```python
from build123d import *

# Parameters (mm, degrees)
RESSALTO_EXTRUS_O1_DEPTH    = 285
CORTE_EXTRUS_O1_DEPTH       = 286
RESSALTO_EXTRUS_O3_DEPTH    = 285
ESBO_O13_W                  = 1.5
ESBO_O13_H                  = 2
CORTE_EXTRUS_O7_DEPTH       = 52.25
CORTE_EXTRUS_O7_DEPTH_BACK  = 52.25
RESSALTO_EXTRUS_O5_DEPTH    = 10
ESBO_O5_R                   = 1.25
CORTE_EXTRUS_O3_DEPTH       = 10
ESBO_O6_W                   = 10
ESBO_O6_H                   = 6.190700041
RESSALTO_EXTRUS_O4_DEPTH    = 11
ESBO_O7_R                   = 2.25
CORTE_EXTRUS_O4_DEPTH       = 12
ESBO_O9_R                   = 1.65
CORTE_EXTRUS_O5_DEPTH       = 10
RESSALTO_EXTRUS_O6_DEPTH    = 15
ESBO_O12_R                  = 2.5
CORTE_EXTRUS_O8_DEPTH       = 20
CORTE_EXTRUS_O9_START       = -11
ESBO_O14_R                  = 6
CORTE_EXTRUS_O9_DEPTH       = 100
PADR_O_LINEAR1_COUNT        = 2
PADR_O_LINEAR1_PITCH        = 230
ESBO_O16_W                  = 118.931950447
ESBO_O16_H                  = 98.407051197
ESBO_O16_W_2                = 168.047643727
ESBO_O16_H_2                = 92.783791129
CORTE_EXTRUS_O11_DEPTH      = 55.553847577
CORTE_EXTRUS_O11_DEPTH_BACK = 55.603847577


with BuildPart() as part:
    # Esbo_o1 → Ressalto-extrus_o1 (new body)
    with BuildSketch(Plane.XY):
        Polygon((-46.053847577, 79.767603888), (-51.25, 88.767603888), (-48.82913331, 88.767603888), (-47.882520117, 115.87505904), (-45.882520117, 115.87505904), (-44.935906924, 88.767603888), (-41.435906924, 88.767603888), (-40.393073045, 118.630458973), (-38.393073045, 118.630458973), (-37.350239166, 88.767603888), (-33.850239166, 88.767603888), (-32.727930438, 120.906320886), (-30.727930438, 120.906320886), (-29.60562171, 88.767603888), (-26.10562171, 88.767603888), (-24.921032923, 122.689788425), (-22.921032923, 122.689788425), (-21.736444137, 88.767603888), (-18.236444137, 88.767603888), (-17.007119627, 123.970851902), (-15.007119627, 123.970851902), (-13.777795118, 88.767603888), (-10.277795118, 88.767603888), (-9.021529135, 124.742354757), (-7.021529135, 124.742354757), (-5.765263153, 88.767603888), (-2.265263153, 88.767603888), (-1, 125), (1, 125), (2.265263153, 88.767603888), (5.765263153, 88.767603888), (7.021529135, 124.742354757), (9.021529135, 124.742354757), (10.277795118, 88.767603888), (13.777795118, 88.767603888), (15.007119627, 123.970851902), (17.007119627, 123.970851902), (18.236444137, 88.767603888), (21.736444137, 88.767603888), (22.921032923, 122.689788425), (24.921032923, 122.689788425), (26.10562171, 88.767603888), (29.60562171, 88.767603888), (30.727930438, 120.906320886), (32.727930438, 120.906320886), (33.850239166, 88.767603888), (37.350239166, 88.767603888), (38.393073045, 118.630458973), (40.393073045, 118.630458973), (41.435906924, 88.767603888), (44.935906924, 88.767603888), (45.882520117, 115.87505904), (47.882520117, 115.87505904), (48.82913331, 88.767603888), (51.25, 88.767603888), (46.053847577, 79.767603888), align=None)
    extrude(amount=RESSALTO_EXTRUS_O1_DEPTH)

    # Esbo_o2 → Corte-extrus_o1 (cut, through all)
    with BuildSketch(Plane.XY.offset(285)):
        Polygon((-47.003847577, 81.413052155), (-43.972758664, 83.163052155), (-45.072758664, 85.068308043), (-48.103847577, 83.318308043), align=None)
    extrude(amount=-CORTE_EXTRUS_O1_DEPTH, mode=Mode.SUBTRACT)


with BuildPart() as body_2:
    # Esbo_o3 → Ressalto-extrus_o3 (new body)
    with BuildSketch(Plane.XY.offset(285)):
        Polygon((47.053847577, 81.499654695), (48.053847577, 83.231705503), (49.785898385, 82.231705503), (48.785898385, 80.499654695), align=None)
    extrude(amount=-RESSALTO_EXTRUS_O3_DEPTH)


with BuildPart() as corte_extrus_o7_tool:
    # Esbo_o13 → Corte-extrus_o7 (new body, two sides)
    with BuildSketch(Plane(origin=(0, 0, 0), x_dir=(0, 0, -1), z_dir=(1, 0, 0))) as corte_extrus_o7_sk:
        with Locations((-284.25, 82.767603888)):
            Rectangle(ESBO_O13_W, ESBO_O13_H)
    extrude(amount=CORTE_EXTRUS_O7_DEPTH)
    extrude(corte_extrus_o7_sk.sketch, amount=-CORTE_EXTRUS_O7_DEPTH_BACK)


with BuildPart() as part_1:
    add(part.part)

    # Corte-extrus_o7: cut by corte_extrus_o7_tool
    add(corte_extrus_o7_tool.part, mode=Mode.SUBTRACT)



with BuildPart() as body_2_1:
    add(body_2.part)

    # Corte-extrus_o7: cut by corte_extrus_o7_tool
    add(corte_extrus_o7_tool.part, mode=Mode.SUBTRACT)


with BuildPart() as part_2:
    add(part_1.part)

    add(body_2_1.part)  # Ressalto-extrus_o5 merges body 2
    # Esbo_o8 → Ressalto-extrus_o5 (add)
    with BuildSketch(Plane(origin=(0, 0, 0), x_dir=(0, 0, -1), z_dir=(0.866025404, -0.5, 0))):
        with BuildLine():
            Line((-280, 104.107695155), (-280, 96.107695155))
            Line((-280, 96.107695155), (-270, 96.107695155))
            Line((-270, 96.107695155), (-270, 104.107695155))
            ThreePointArc((-270, 104.107695155), (-275, 109.107695155), (-280, 104.107695155))
        make_face()
    ressalto_extrus_o5 = extrude(amount=-RESSALTO_EXTRUS_O5_DEPTH)

    # Esbo_o5 → Corte-extrus_o3 (cut)
    with BuildSketch(Plane.XY.offset(285)):
        with Locations((-30, 85.267603888)):
            Circle(ESBO_O5_R)
        with Locations((30, 85.267603888)):
            Circle(ESBO_O5_R)
    extrude(amount=-CORTE_EXTRUS_O3_DEPTH, mode=Mode.SUBTRACT)

    # Esbo_o6 → Ressalto-extrus_o4 (add)
    with BuildSketch(Plane(origin=(0, 0, 0), x_dir=(0, 0, 1), z_dir=(-0.866025404, -0.5, 0))):
        with BuildLine():
            Line((280, 102.5), (280, 104.207693629))
            ThreePointArc((280, 104.207693629), (275, 109.207695155), (270, 104.207693629))
            Line((270, 104.207693629), (270, 102.5))
            Line((270, 102.5), (280, 102.5))
        make_face()
        with Locations((275, 99.404649979)):
            Rectangle(ESBO_O6_W, ESBO_O6_H)
    ressalto_extrus_o4 = extrude(amount=-RESSALTO_EXTRUS_O4_DEPTH)

    # Esbo_o7 → Corte-extrus_o4 (cut)
    with BuildSketch(Plane(origin=(0, 0, 0), x_dir=(0, 0, 1), z_dir=(-0.866025404, -0.5, 0))):
        with Locations((275, 104.207695155)):
            Circle(ESBO_O7_R)
    corte_extrus_o4 = extrude(amount=-CORTE_EXTRUS_O4_DEPTH, mode=Mode.SUBTRACT)

    # Esbo_o9 → Corte-extrus_o5 (cut)
    with BuildSketch(Plane(origin=(0, 0, 0), x_dir=(0, 0, -1), z_dir=(0.866025404, -0.5, 0))):
        with Locations((-275, 104.107695155)):
            Circle(ESBO_O9_R)
    corte_extrus_o5 = extrude(amount=-CORTE_EXTRUS_O5_DEPTH, mode=Mode.SUBTRACT)

    # Esbo_o10 → Ressalto-extrus_o6 (add)
    with BuildSketch(Plane(origin=(0, 0, 0), x_dir=(-1, 0, 0), z_dir=(0, 0, -1))):
        Polygon((5.765263153, 88.767603888), (6.680885729, 114.987603888), (1.349640577, 114.987603888), (2.265263153, 88.767603888), align=None)
        Polygon((-2.265263153, 88.767603888), (-1.349640577, 114.987603888), (-6.680885729, 114.987603888), (-5.765263153, 88.767603888), align=None)
    extrude(amount=-RESSALTO_EXTRUS_O6_DEPTH)

    # Esbo_o12 → Corte-extrus_o8 (cut)
    with BuildSketch(Plane(origin=(0, 0, 0), x_dir=(-1, 0, 0), z_dir=(0, 0, -1))):
        with Locations((0, 104.999999962)):
            Circle(ESBO_O12_R)
    extrude(amount=-CORTE_EXTRUS_O8_DEPTH, mode=Mode.SUBTRACT)

    # Esbo_o14 → Corte-extrus_o9 (cut)
    with BuildSketch(Plane(origin=(0, 0, 0), x_dir=(0, 0, 1), z_dir=(-0.866025404, -0.5, 0)).offset(CORTE_EXTRUS_O9_START)):
        with Locations((275, 104.207695155)):
            Circle(ESBO_O14_R)
    corte_extrus_o9 = extrude(amount=-CORTE_EXTRUS_O9_DEPTH, mode=Mode.SUBTRACT)

    # Padr_o linear1: Ressalto-extrus_o5, Ressalto-extrus_o4, Corte-extrus_o4, Corte-extrus_o5, Corte-extrus_o9 ×2
    with Locations(*[(0, 0, -i * PADR_O_LINEAR1_PITCH) for i in range(1, PADR_O_LINEAR1_COUNT)]):
        add(ressalto_extrus_o5)
        add(ressalto_extrus_o4)
        add(corte_extrus_o4, mode=Mode.SUBTRACT)
        add(corte_extrus_o5, mode=Mode.SUBTRACT)
        add(corte_extrus_o9, mode=Mode.SUBTRACT)

    # Esbo_o16 → Corte-extrus_o11 (cut, two sides)
    with BuildSketch(Plane(origin=(0, 0, 0), x_dir=(0, 0, -1), z_dir=(1, 0, 0))) as corte_extrus_o11_sk:
        with Locations((-250.695007134, 104.881737693)):
            Rectangle(ESBO_O16_W, ESBO_O16_H)
        with Locations((-57.205210046, 102.070107659)):
            Rectangle(ESBO_O16_W_2, ESBO_O16_H_2)
    extrude(amount=CORTE_EXTRUS_O11_DEPTH, mode=Mode.SUBTRACT)
    extrude(corte_extrus_o11_sk.sketch, amount=-CORTE_EXTRUS_O11_DEPTH_BACK, mode=Mode.SUBTRACT)


solid = part_2.part
```
Geometry: final body of the model. Coordinates: model frame, mm. A direction names the side the tool comes from. Round coordinates to 2 decimals unless told otherwise and drop trailing zeros. Write each loop counter-clockwise with the first axis right and the second up, starting at its lowest first coordinate (ties: lowest second). Pieces come first, ordered by that corner, then holes. Notation, with made-up numbers: M -11,22.25 L 21,22.25 A7 ccw 21,34.25 Z; hole C 1.25,10 d8. An arc over 180 degrees is marked long. Answer in a Markdown table with one row per item. Add a question column.
(1) Reachability of faces 5 (the face through (-4, 88.768, 166)), 6 (the face through (50, 88.768, 166)), 7 (the face through (-32, 120.906, 166)) from +Z, -Z, +X, -X, +Y, -Y: full face, straight path, thin tool, end or side. Return the list, or none.
(2) Cut plane A-A, the plane x = -20. Return the cut outline in (y, z), then the cut area to 3 significant figures.
(3) Ray query, L1, parallel to Y at x = 12, z = 174.5; L2, parallel to Y at x = -7.5, z = 148. Return the intervals inside material, ascending.
(4) Draft query along X for faces 1 (the face through (47, 115.875, 166)), 2 (the face through (-49.65, 86, 165.88)), 3 (the face through (4, 88.768, 166)), 4 (the face through (36, 88.768, 166)). Return one class per face: pulls with the +X half, pulls with the -X half, needs draft (parallel to the pull), parting line crosses it, or undercut.
(5) Cut plane B-B, the plane y = 114. Give the number of separate pieces and of enclosed holes in the cut face, then the cut area to 3 significant figures.
(6) Cut plane C-C, the plane y = 87. Return the cut outline in (x, z), then the cut area to 3 significant figures.
(7) Contact query for flat-ended pins moving along their axis: pin 1 (1 mm diameter, centred on x = -31.5, z = 170, fed in from +Y); pin 2 (1 mm diameter, centred on x = -35.5, z = 178.5, fed in from +Y); pin 3 (12 mm diameter, centred on x = -27.5, y = 103.5, fed in from +Z); pin 4 (12 mm diameter, centred on y = 93.5, z = 177.5, fed in from -X). Output: stop coordinate, or through.
Established:
| question | item | result |
|---|---|---|
| 1 | face 5 | +Z, -Z, +Y |
| 1 | face 6 | +Z, -Z, +X, +Y |
| 1 | face 7 | +Z, -Z, -X, +Y |
| 2 | outline | M 79.77,141.23 L 88.77,141.23 L 88.77,191.23 L 79.77,191.23 Z |
| 2 | area | 450 mm² |
| 3 | L1 | 79.77 to 88.77 |
| 3 | L2 | 79.77 to 124.74 |
| 4 | face 1 | needs draft |
| 4 | face 2 | pulls with the -X half |
| 4 | face 3 | undercut |
| 4 | face 4 | undercut |
| 5 | separate pieces | 13 |
| 5 | enclosed holes | 0 |
| 5 | area | 1,640 mm² |
| 6 | outline | M -50.23,141.23 L 50.23,141.23 L 50.23,191.23 L -50.23,191.23 Z |
| 6 | area | 5,020 mm² |
| 7 | pin 1 | y = 120.91 |
| 7 | pin 2 | y = 88.77 |
| 7 | pin 3 | z = 191.23 |
| 7 | pin 4 | x = -51.25 |
